Part model, mm, in its own coordinate system. A direction names the side the tool comes from. Round coordinates to 2 decimals unless told otherwise and drop trailing zeros. Order: outer loops, then holes, each group sorted by start corner. A loop starts at its lowest first (then second) coordinate and runs counter-clockwise, first axis right, second up. Notation, with made-up numbers: M -10,37 L 0,37 A19 ccw 0,68 Z; hole C 57.25,8.25 d9. An arc over 180 degrees is marked long. Write each question's results on one line, items separated by ' | '. Start each with the question number.
1. Band-saw the part on B-B, the plane y = -12.5. List the corners of the cut face in (x, z).
2. Two-plate mould, pull along Y, no slides. Class faces 1 (the face through (0, -15, 5)), 2 (the face through (0, 13, 15)), 3 (the face through (-2, 4, 12)), 4 (the face through (1.5, -6, 14)): +Y half, -Y half, draft (parallel to the pull), parting line (faces both ways), or undercut.
3. Band-saw the part on A-A, the plane x = -5.25. List the corners of the cut face in (y, z).
4. Which spindle directions (+Z, -Z, +X, -X, +Y, -Y) get a long thin tool onto all of the face, cutting with end or side? Do faces 5 (the face through (0.08, 0.63, 14.87)), 6 (the face through (6, 6, 14)), 7 (the face through (-0.08, -0.35, 14.68)), 8 (the face through (0.021, -3.414, 14.09)), 9 (the face through (-0.021, -9.306, 12.957)). Say none if no direction does.
5. Probe L1, parallel to Z at x = -5, y = 2.25; L2, parallel to Z at x = 7, y = 9; L3, parallel to X at y = 3, z = 13.25. List the from-to ranges inside material, lowest first. Write a range as [from, to].
6. Drop flat-ended pins along their axis: pin 1 Ø1 at (x, y) = (-3.5, 4.5) entering from -Z; pin 2 Ø2.5 at (y, z) = (-6, 15.5) entering from +X; pin 3 Ø2.5 at (y, z) = (-6, 15) entering from -X; pin 4 Ø2.5 at (x, z) = (-1, 14.5) entering from +Y. Give the stop position or say it passes through.
7. Band-saw the part on C-C, the plane y = -6.25. List the corners of the cut face in (x, z).
```python
from build123d import *

# Parameters (mm, degrees)
CROQUIS1_W              = 15
CROQUIS1_H              = 30
SALIENTE_EXTRUIR1_DEPTH = 10
CROQUIS2_R              = 3.75
SALIENTE_EXTRUIR2_DEPTH = 2
CROQUIS3_W              = 15
CROQUIS3_H              = 30
SALIENTE_EXTRUIR3_DEPTH = 1
CROQUIS4_W              = 12
CROQUIS4_H              = 26
SALIENTE_EXTRUIR4_DEPTH = 5
CORTAR_EXTRUIR1_DEPTH   = 12
CORTAR_EXTRUIR2_DEPTH   = 1.5


with BuildPart() as part:
    # Croquis1 → Saliente-Extruir1 (new body)
    with BuildSketch(Plane.XY):
        Rectangle(CROQUIS1_W, CROQUIS1_H)
    extrude(amount=SALIENTE_EXTRUIR1_DEPTH)

    # Croquis2 → Saliente-Extruir2 (add)
    with BuildSketch(Plane.XY.offset(10)):
        with Locations(Location((0, 0, 0), (0, 0, 180))):
            Circle(CROQUIS2_R)
    extrude(amount=SALIENTE_EXTRUIR2_DEPTH)

    # Croquis3 → Saliente-Extruir3 (add)
    with BuildSketch(Plane.XY.offset(12)):
        Rectangle(CROQUIS3_W, CROQUIS3_H)
    extrude(amount=SALIENTE_EXTRUIR3_DEPTH)

    # Croquis4 → Saliente-Extruir4 (add)
    with BuildSketch(Plane.XY.offset(13)):
        Rectangle(CROQUIS4_W, CROQUIS4_H)
    extrude(amount=SALIENTE_EXTRUIR4_DEPTH)

    # Croquis5 → Cortar-Extruir1 (cut)
    with BuildSketch(Plane(origin=(6, 0, 0), x_dir=(0, 0, -1), z_dir=(1, 0, 0))):
        Polygon((-18, 13), (-13, -13), (-18, -13), align=None)
    extrude(amount=-CORTAR_EXTRUIR1_DEPTH, mode=Mode.SUBTRACT)

    # Croquis6 → Cortar-Extruir2 (cut)
    with BuildSketch(Plane(origin=(0, -2.87446505, 14.94721826), x_dir=(1, 0, 0), z_dir=(0, -0.18884739365012454, 0.9820064469806473))):
        with BuildLine():
            ThreePointArc((-2.350627634, 12.139409427), (-3.5, 9.546235749), (-2.350627634, 6.953062071))
            Line((-2.350627634, 6.953062071), (-1.846921712, 7.508742145))
            ThreePointArc((-1.846921712, 7.508742145), (-2.75, 9.546235749), (-1.846921712, 11.583729353))
            Line((-1.846921712, 11.583729353), (-2.350627634, 12.139409427))
        make_face()
        with BuildLine():
            Line((-1.846921712, 7.508742145), (-2.350627634, 6.953062071))
            ThreePointArc((-2.350627634, 6.953062071), (0, 6.046235749), (2.350627634, 6.953062071))
            Line((2.350627634, 6.953062071), (1.846921712, 7.508742145))
            ThreePointArc((1.846921712, 7.508742145), (0, 6.796235749), (-1.846921712, 7.508742145))
        make_face()
        with BuildLine():
            Line((1.846921712, 7.508742145), (2.350627634, 6.953062071))
            ThreePointArc((2.350627634, 6.953062071), (3.199780986, 8.127996827), (3.5, 9.546235749))
            ThreePointArc((3.5, 9.546235749), (3.199780986, 10.964474671), (2.350627634, 12.139409427))
            Line((2.350627634, 12.139409427), (1.846921712, 11.583729353))
            ThreePointArc((1.846921712, 11.583729353), (2.514113632, 10.660566331), (2.75, 9.546235749))
            ThreePointArc((2.75, 9.546235749), (2.514113632, 8.431905167), (1.846921712, 7.508742145))
        make_face()
        with BuildLine():
            ThreePointArc((2.350627634, 12.139409427), (0, 13.046235749), (-2.350627634, 12.139409427))
            Line((-2.350627634, 12.139409427), (-1.846921712, 11.583729353))
            ThreePointArc((-1.846921712, 11.583729353), (0, 12.296235749), (1.846921712, 11.583729353))
            Line((1.846921712, 11.583729353), (2.350627634, 12.139409427))
        make_face()
        Polygon((-1.5, -0.691966546), (-1.5, -2.037191259), (0, -3.691966546), (1.5, -2.037191259), (1.5, -0.691966546), align=None)
        Polygon((0, -3.691966546), (-1.5, -5.346741833), (-1.5, -6.691966546), (1.5, -6.691966546), (1.5, -5.346741833), align=None)
        Polygon((1.5, -5.346741833), (1.5, -2.037191259), (0, -3.691966546), align=None)
        Polygon((0, -3.691966546), (-1.5, -2.037191259), (-1.5, -5.346741833), align=None)
        Polygon((-5.546766255, 3.427134602), (-6, 2.927134602), (6, 2.927134602), (5.546766255, 3.427134602), align=None)
        Polygon((6, 2.927134602), (-6, 2.927134602), (-5.546766255, 2.427134602), (5.546766255, 2.427134602), align=None)
        Polygon((5.546766255, 3.427134602), (6, 2.927134602), (6, 3.427134602), align=None)
        Polygon((6, 2.427134602), (6, 2.927134602), (5.546766255, 2.427134602), align=None)
        Polygon((-6, 3.427134602), (-6, 2.927134602), (-5.546766255, 3.427134602), align=None)
        Polygon((-5.546766255, 2.427134602), (-6, 2.927134602), (-6, 2.427134602), align=None)
    extrude(amount=-CORTAR_EXTRUIR2_DEPTH, mode=Mode.SUBTRACT)


solid = part.part
```
Solution:
1) outline: M -7.5,0 L 7.5,0 L 7.5,10 L -7.5,10 Z; M -7.5,12 L 7.5,12 L 7.5,13 L 6,13 L 6,13.1 L -6,13.1 L -6,13 L -7.5,13 Z
2) face 1: -Y half | face 2: +Y half | face 3: draft | face 4: undercut
3) outline: M -15,0 L 15,0 L 15,10 L -15,10 Z; M -15,12 L 15,12 L 15,13 L 13,13 L 13,18 L 0.49,15.59 L 0.77,14.12 L -0.21,13.93 L -0.49,15.41 L -13,13 L -15,13 Z
4) face 5: +X, -X | face 6: +Z, +X, +Y, -Y | face 7: +Z, +X, -X | face 8: none | face 9: +Z
5) L1: [0, 10], [12, 15.93] | L2: [0, 10], [12, 13] | L3: [-6, 6]
6) pin 1: z = 0 | pin 2: x = 6 | pin 3: x = -6 | pin 4: y = 13
7) outline: M -7.5,0 L 7.5,0 L 7.5,10 L -7.5,10 Z; M -7.5,12 L 7.5,12 L 7.5,13 L 6,13 L 6,14.3 L 1.5,14.3 L 1.5,12.77 L -1.5,12.77 L -1.5,14.3 L -6,14.3 L -6,13 L -7.5,13 Z
